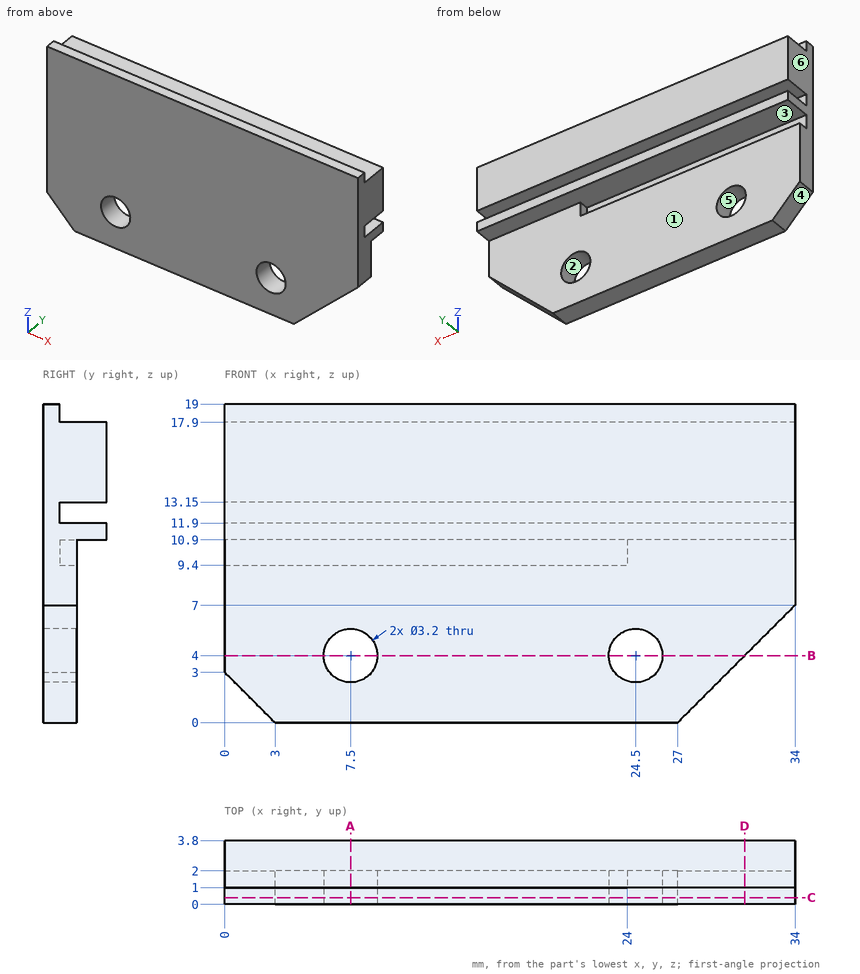
Input: dimensioned drawing with shaded views. Units: mm. Origin: part minimum x, y, z. A direction names the side the tool comes from. Coordinates: 2 decimals unless noted, no trailing zeros. Order: outer loops, then holes, each group sorted by start corner. A loop starts at its lowest first (then second) coordinate and runs counter-clockwise, first axis right, second up. Notation, with made-up numbers: (9, 7.5) -> (65, 7.5) arc R13 cw to (65, 19.5) -> close; hole circle Ø10 at (-9.5, 75.5). An arc over 180 degrees is marked (long way). Answer in a Markdown table with one row per item.
Item 1: Section B-B on z = 4. Output: boundary loops of the cut face in (x, y).
Return value:
| item | result |
|---|---|
| outline | (0, 0) -> (5.9, 0) -> (5.9, 2) -> (0, 2) -> close; (9.1, 0) -> (22.9, 0) -> (22.9, 2) -> (9.1, 2) -> close; (26.1, 0) -> (31, 0) -> (31, 2) -> (26.1, 2) -> close |
Item 2: Draft query along Z for the marked faces 4, 5 and 6. Return one class per face: released by +Z, released by -Z, zero draft, split by the parting line, or undercut.
Return value:
| item | result |
|---|---|
| face 4 | released by -Z |
| face 5 | undercut |
| face 6 | zero draft |
Item 3: Ray query, L1, parallel to Z at x = 13.5, y = 1.55; L2, parallel to Z at x = 18, y = 2.1; L3, parallel to X at y = 1.4, z = 3.25. Return the intervals inside material, ascending.
Return value:
| item | result |
|---|---|
| L1 | z = 0 to 9.4, 10.9 to 11.9, 13.15 to 17.9 |
| L2 | z = 10.9 to 11.9, 13.15 to 17.9 |
| L3 | x = 0 to 6.09, 8.91 to 23.09, 25.91 to 30.25 |
Item 4: Section D-D on x = 31. Output: boundary loops of the cut face in (y, z).
Return value:
| item | result |
|---|---|
| outline | (0, 4) -> (2, 4) -> (2, 10.9) -> (3.8, 10.9) -> (3.8, 11.9) -> (1, 11.9) -> (1, 13.15) -> (3.8, 13.15) -> (3.8, 17.9) -> (1, 17.9) -> (1, 19) -> (0, 19) -> close |
Item 5: Section C-C on y = 0.4. Output: boundary loops of the cut face in (x, z), plus the area to 3 significant figures.
Return value:
| item | result |
|---|---|
| outline | (0, 3) -> (3, 0) -> (27, 0) -> (34, 7) -> (34, 19) -> (0, 19) -> close; hole circle Ø3.2 at (7.5, 4); hole circle Ø3.2 at (24.5, 4) |
| area | 601 mm² |
Item 6: Access query for the marked faces 1, 2 and 3. Directions: +Z, -Z, +X, -X, +Y, -Y. A direction counts if a zero-diameter tool reaches every point of the face in a straight line with its end or side. Return the directions, or none.
Return value:
| item | result |
|---|---|
| face 1 | -Z, +X, -X, +Y |
| face 2 | +Y, -Y |
| face 3 | -X, +Y |
Item 7: Contact query for flat-ended pins moving along their axis: P1, Ø5, axis at x = 7.5, z = 4, coming from the +Y side; P2, Ø1, axis at x = 19, z = 12.5, coming from the +Y side; P3, Ø0.5, axis at y = 1.5, z = 10, coming from the -X side. Output: stop coordinate, or through.
Return value:
| item | result |
|---|---|
| P1 | stops at y = 2 |
| P2 | stops at y = 1 |
| P3 | stops at x = 24 |
Item 8: Section A-A on x = 7.5. Output: boundary loops of the cut face in (y, z).
Return value:
| item | result |
|---|---|
| outline | (0, 0) -> (2, 0) -> (2, 2.4) -> (0, 2.4) -> close; (0, 5.6) -> (2, 5.6) -> (2, 9.4) -> (1, 9.4) -> (1, 10.9) -> (3.8, 10.9) -> (3.8, 11.9) -> (1, 11.9) -> (1, 13.15) -> (3.8, 13.15) -> (3.8, 17.9) -> (1, 17.9) -> (1, 19) -> (0, 19) -> close |
